Design review of the part built by this model. Coordinates are the model's own, in mm. Face numbers are marked on the shaded views. Coordinates: 2 decimals unless noted, no trailing zeros. Order: outer loops, then holes, each group sorted by start corner. A loop starts at its lowest first (then second) coordinate and runs counter-clockwise, first axis right, second up. Notation, with made-up numbers: M -13,43 L 36,43 A34 ccw 36,73 Z; hole C 56.25,-19 d7. An arc over 180 degrees is marked long. Answer as a JSON object with one key per item and string values.
from build123d import *

# Parameters (mm, degrees)
SKETCH1_R                      = 11.1125
BOSS_EXTRUDE1_DEPTH            = 19.05
F_1_2_0_5_DIAMETER_HOLE1_D     = 12.7
F_1_2_0_5_DIAMETER_HOLE1_DEPTH = 22.352
F_1_2_0_5_DIAMETER_HOLE1_TIP   = 3.815464931
SKETCH10_R                     = 3.2639
CUT_EXTRUDE3_DEPTH             = 42.21389708


with BuildPart() as part:
    # Sketch1 → Boss-Extrude1 (new, symmetric)
    with BuildSketch(Plane.XY):
        with Locations(Location((0, 0, 0), (0, 0, 180))):
            Circle(SKETCH1_R)
    extrude(amount=BOSS_EXTRUDE1_DEPTH, both=True)

    # 1/2 (0.5) Diameter Hole1
    with Locations(Plane.XY.offset(19.05)):
        with Locations((0, 0)):
            Hole(F_1_2_0_5_DIAMETER_HOLE1_D / 2, depth=F_1_2_0_5_DIAMETER_HOLE1_DEPTH)
            with Locations((0, 0, -(F_1_2_0_5_DIAMETER_HOLE1_DEPTH + F_1_2_0_5_DIAMETER_HOLE1_TIP / 2))):  # 118° drill point
                Cone(0, F_1_2_0_5_DIAMETER_HOLE1_D / 2, F_1_2_0_5_DIAMETER_HOLE1_TIP, mode=Mode.SUBTRACT)

    # Sketch10 → Cut-Extrude3 (cut, through all)
    with BuildSketch(Plane.XY.offset(19.05)):
        Circle(SKETCH10_R)
    extrude(amount=-CUT_EXTRUDE3_DEPTH, mode=Mode.SUBTRACT)


solid = part.part
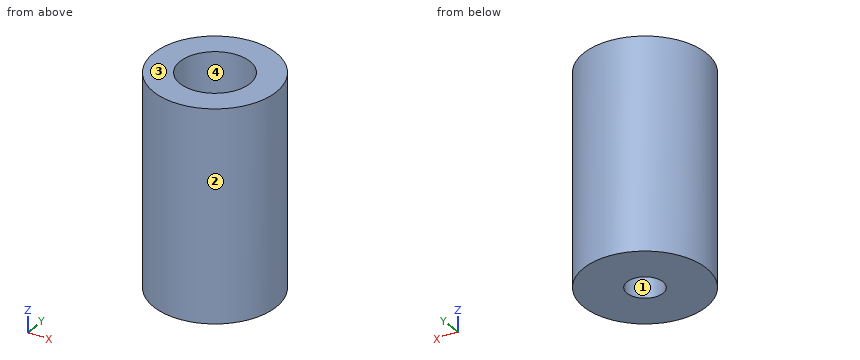
1) Add section D-D (z = -7). State the section outline as (x, y) points (1 decimal).
Taken from the geometry:
{"outline": "C 0,0 d22.2; hole C 0,0 d6.5"}
2) To check wall thickness, follow L1, parallel to X at y = -3.75, z = 4.5; L2, parallel to Y at x = 0, z = -7.75; L3, parallel to Y at x = 0, z = 8. State the ranges of each line that lie inside material, in increasing order.
Taken from the geometry:
{"L1": "x = -10.46 to -5.12, 5.12 to 10.46", "L2": "y = -11.11 to -3.26, 3.26 to 11.11", "L3": "y = -11.11 to -6.35, 6.35 to 11.11"}
3) Mouldability with a two-part tool opening along Y and no side actions: class the marked faces 1, 2, 3 and 4 as released by +Y, released by -Y, zero draft, split by the parting line, or undercut.
Taken from the geometry:
{"face 1": "undercut", "face 2": "split by the parting line", "face 3": "zero draft", "face 4": "undercut"}
4) Insertion check: pin 1 Ø1 at (x, z) = (-5.5, -3) entering from -Y; pin 2 Ø5 at (x, z) = (6, -2.5) entering from -Y; pin 3 Ø2 at (y, z) = (-6, -9.5) entering from +X. Each pin has a flat end and moves straight along its axis. Give the tip position at first contact, or say it passes through.
Taken from the geometry:
{"pin 1": "stops at y = -9.92", "pin 2": "stops at y = -10.55", "pin 3": "stops at x = 9.92"}
5) Add section A-A (x = 0). State the section outline as (y, z) points, and give its area (3 significant figures).
Taken from the geometry:
{"outline": "M -11.11,-19.05 L -3.26,-19.05 L -3.26,-5.16 L -6.35,-3.3 L -6.35,19.05 L -11.11,19.05 Z; M 3.26,-19.05 L 11.11,-19.05 L 11.11,19.05 L 6.35,19.05 L 6.35,-3.3 L 3.26,-5.16 Z", "area": "454 mm2"}
